```python
from build123d import *

# Parameters (mm, degrees)
CROQUIS1_R              = 25.4
SALIENTE_EXTRUIR1_DEPTH = 12.7
SALIENTE_EXTRUIR2_REACH = 68.04
CROQUIS2_R              = 12.7
CROQUIS3_R              = 16.51
SALIENTE_EXTRUIR3_DEPTH = 7.62
CROQUIS4_R              = 19.05
SALIENTE_EXTRUIR4_DEPTH = 5.08
CROQUIS6_R              = 6.35
SALIENTE_EXTRUIR5_DEPTH = 34.29


with BuildPart() as part:
    # Croquis1 → Saliente-Extruir1 (new body, symmetric)
    with BuildSketch(Plane(origin=(0, 0, 0), x_dir=(0, 0, -1), z_dir=(1, 0, 0))):
        Circle(CROQUIS1_R)
    extrude(amount=SALIENTE_EXTRUIR1_DEPTH, both=True)

    # Croquis2 → Saliente-Extruir2 (add, up to next)
    with BuildSketch(Plane.XY.offset(40.64), mode=Mode.PRIVATE) as saliente_extruir2_sk1:
        Circle(CROQUIS2_R)
    saliente_extruir2_tool1 = extrude(saliente_extruir2_sk1.sketch, amount=-SALIENTE_EXTRUIR2_REACH, mode=Mode.PRIVATE) - part.part
    add(saliente_extruir2_tool1.solids().sort_by_distance((0, 0, 40.64))[0])

    # Croquis3 → Saliente-Extruir3 (add)
    with BuildSketch(Plane.XY.offset(40.64)):
        Circle(CROQUIS3_R)
    extrude(amount=SALIENTE_EXTRUIR3_DEPTH)

    # Croquis4 → Saliente-Extruir4 (add)
    with BuildSketch(Plane.XY.offset(48.26)):
        Circle(CROQUIS4_R)
    extrude(amount=SALIENTE_EXTRUIR4_DEPTH)

    # Croquis6 → Saliente-Extruir5 (add, symmetric)
    with BuildSketch(Plane(origin=(0, 0, 0), x_dir=(0, 0, -1), z_dir=(1, 0, 0))):
        Circle(CROQUIS6_R)
    extrude(amount=SALIENTE_EXTRUIR5_DEPTH, both=True)


solid = part.part
```
The model under review builds one solid part; all positions refer to its coordinate system, in mm. A direction names the side the tool comes from. Coordinates: 2 decimals unless noted, no trailing zeros. Write each loop counter-clockwise with the first axis right and the second up, starting at its lowest first coordinate (ties: lowest second). Pieces come first, ordered by that corner, then holes. Notation, with made-up numbers: (43.5, 58) - (63.5, 58) arc R16 ccw to (63.5, 63) - close; hole circle Ø8 at (54.25, 39.5). An arc over 180 degrees is marked (long way). Write item = value, one per line.
(1) Consider section A-A, the plane z = 0. Give the boundary of the cut face in (x, y).
Result sheet:
outline = (-34.29, -6.35) - (-12.7, -6.35) - (-12.7, -25.4) - (12.7, -25.4) - (12.7, -6.35) - (34.29, -6.35) - (34.29, 6.35) - (12.7, 6.35) - (12.7, 25.4) - (-12.7, 25.4) - (-12.7, 6.35) - (-34.29, 6.35) - close
(2) Consider section C-C, the plane x = -14. Give the boundary of the cut face in (y, z).
Result sheet:
outline = (-12.92, 48.26) - (-8.75, 48.26) - (-8.75, 40.64) - (8.75, 40.64) - (8.75, 48.26) - (12.92, 48.26) - (12.92, 53.34) - (-12.92, 53.34) - close; circle Ø12.7 at (0, 0)
(3) Machinability: for faces 1 (the face through (23.65, -6.2, 1.38)), 2 (the face through (-23.34, -6.2, 1.38)), 3 (the face through (-6, 16, 48.26)), which of the approach directions +Z, -Z, +X, -X, +Y, -Y give a long, thin tool a straight path to every point of the face, cutting with its end or side? Answer none if there is none.
Result sheet:
face_1 = +X
face_2 = -X
face_3 = none
(4) For P1, Ø6, axis at y = 12.5, z = 30.5, coming from the +X side; P2, Ø19, axis at x = -7, y = -7, coming from the -Z side; P3, Ø10, axis at x = -23, y = 3.5, coming from the -Z side; P4, Ø1, axis at x = -12.5, z = 17, coming from the -Y side, all flat-tipped, find the tip position at first contact; note any pin that passes through.
Result sheet:
P1 = 8.43
P2 = -25.4
P3 = -6.35
P4 = -19.31
(5) Consider section B-B, the plane x = 0. Give the boundary of the cut face in (y, z), then the cut area to 3 significant figures.
Result sheet:
outline = (-19.05, 48.26) - (-16.51, 48.26) - (-16.51, 40.64) - (-12.7, 40.64) - (-12.7, 22) arc R25.4 ccw (long way) to (12.7, 22) - (12.7, 40.64) - (16.51, 40.64) - (16.51, 48.26) - (19.05, 48.26) - (19.05, 53.34) - (-19.05, 53.34) - close
area = 2,890 mm^2
(6) Consider section D-D, the plane y = -8. Give the boundary of the cut face in (x, z).
Result sheet:
outline = (-17.29, 48.26) - (-14.44, 48.26) - (-14.44, 40.64) - (-9.86, 40.64) - (-9.86, 24.11) - (-12.7, 24.11) - (-12.7, -24.11) - (12.7, -24.11) - (12.7, 24.11) - (9.86, 24.11) - (9.86, 40.64) - (14.44, 40.64) - (14.44, 48.26) - (17.29, 48.26) - (17.29, 53.34) - (-17.29, 53.34) - close
(7) For line 1 (X direction, y = 22.5, z = 5.5); line 2 (Z direction, x = -11.5, y = 13); line 3 (X direction, y = 6, z = 50), list the stretches that pass through material, from the lowest coordinate up. Write a range as [from, to].
Result sheet:
line_1 = [-12.7, 12.7]
line_2 = [-21.82, 21.82], [48.26, 53.34]
line_3 = [-18.08, 18.08]
(8) Mouldability with a two-part tool opening along Z and no side actions: class faces 4 (the face through (0, 0, 53.34)), 5 (the face through (12.7, -5, -5)), 6 (the face through (-34.29, 0, 0)) as pulls with the +Z half, pulls with the -Z half, needs draft (parallel to the pull), parting line crosses it, or undercut.
Result sheet:
face_4 = pulls with the +Z half
face_5 = undercut
face_6 = needs draft
